CAD build for the part. Positions are in the model's coordinates, mm. A direction names the side the tool comes from. Coordinates: 2 decimals unless noted, no trailing zeros. Loops run counter-clockwise (first coordinate to the right, second up) from the corner with the lowest first, then second, coordinate; pieces in that order, holes last. Notation, with made-up numbers: (71, 46.5) -> (128, 46.5) arc R16 cw to (128, 57.5) -> close; hole circle Ø4 at (53, -22.75). An arc over 180 degrees is marked (long way). Write item = value, one per line. Start each with the question number.
(1) Pull direction Z, two halves, no side cores. Call faces 1 (the face through (-5.95, 4.19, -0.13)), 2 (the face through (39.1, 2.5, 13.5)), 3 (the face through (36, 2, 15)), 4 (the face through (-40, 2, 19)): +Z half, -Z half, draft (parallel to the pull), parting line (faces both ways), or undercut.
(2) Band-saw the part on C-C (x = -40). Write the cut outline in (y, z).
(3) Flat gauge pins, fed straight in: P1, Ø3, axis at x = -5.5, y = 4, coming from the +Z side; P2, Ø4.5, axis at x = 40, z = 15, coming from the +Y side; P3, Ø5, axis at x = -2, z = 2.5, coming from the +Y side. Where does each tip first touch, or does it go through?
(4) Band-saw the part on A-A (x = 40). Write the cut outline in (y, z), and give its area (3 significant figures).
(5) Band-saw the part on D-D (z = 0). Write the cut outline in (x, y), and give its area (3 significant figures).
(6) Band-saw the part on B-B (z = 15). Write the cut outline in (x, y), and give its area (3 significant figures).
(7) Tool access for faces 5 (the face through (42, 5, 15)), 6 (the face through (-29.4, 3.5, 0.1)), 7 (the face through (-36, 2, -15)): list every direction of +Z, -Z, +X, -X, +Y, -Y with a clear straight run to the whole face (end or side of a thin tool).
(8) Drill centre lines: line 1 (Z direction, x = 40, y = 1.15); line 2 (X direction, y = 4.25, z = -15.5); line 3 (X direction, y = 1.25, z = 12.5). Where is each one in solid material? Low to high. Write a range as from..to.
Autodesk Inventor part; units mm, degrees
ref_plane "YZ Plane" through (0, 0, 0) normal (1, 0, 0) x (0, 1, 0)
ref_plane "XZ Plane" through (0, 0, 0) normal (0, 1, 0) x (-1, 0, 0)
ref_plane "XY Plane" through (0, 0, 0) normal (0, 0, 1) x (1, 0, 0)
sketch "Sketch1" plane through (0, 0, 0) normal (0, 1, 0) x (-1, 0, 0)
  line L0 (44, 11) -> (-44, 11)
  line L1 (-44, 11) -> (-44, -11)
  line L2 (-44, -11) -> (44, -11)
  line L3 (44, -11) -> (44, 11)
  line L4 (44, 11) -> (-44, -11) construction
  line L5 (-44, 11) -> (44, -11) construction
  line L6 (36, 19) -> (44, 19)
  line L7 (44, 19) -> (44, 11)
  line L8 (44, 11) -> (36, 11)
  line L9 (36, 11) -> (36, 19)
  line L10 (36, 19) -> (44, 11) construction
  line L11 (44, 19) -> (36, 11) construction
  line L12 (36, -19) -> (44, -19)
  line L13 (44, -19) -> (44, -11)
  line L14 (44, -11) -> (36, -11)
  line L15 (36, -11) -> (36, -19)
  line L16 (36, -19) -> (44, -11) construction
  line L17 (44, -19) -> (36, -11) construction
  line L18 (-36, 19) -> (-44, 19)
  line L19 (-44, 19) -> (-44, 11)
  line L20 (-44, 11) -> (-36, 11)
  line L21 (-36, 11) -> (-36, 19)
  line L22 (-36, 19) -> (-44, 11) construction
  line L23 (-44, 19) -> (-36, 11) construction
  line L24 (-36, -19) -> (-44, -19)
  line L25 (-44, -19) -> (-44, -11)
  line L26 (-44, -11) -> (-36, -11)
  line L27 (-36, -11) -> (-36, -19)
  line L28 (-36, -19) -> (-44, -11) construction
  line L29 (-44, -19) -> (-36, -11) construction
  circle A0 centre (40, 15) radius 1.75
  circle A1 centre (40, -15) radius 1.75
  circle A2 centre (-40, 15) radius 1.75
  circle A3 centre (-40, -15) radius 1.75
  point P0 (0, 0)
  dimension "d0" = 22
  dimension "d1" = 88
  dimension "d2" = 8
  dimension "d3" = 8
  dimension "d8" = 3.5
  dimension "d9" = 3.5
  dimension "d10" = 3.5
  dimension "d11" = 3.5
  dimension "d24" = 30
  dimension "d25" = 80
extrude "Extrusion1" add sketch "Sketch1" along normal blind 10 contours L3 L2 L1 L0
extrude "Extrusion2" add sketch "Sketch1" along normal blind 5 contours L0 L9 L6 L7 | L13 L12 L15 L2 | L0 L19 L18 L21 | L27 L24 L25 L2
sketch "Sketch3" plane through (0, 10, 0) normal (0, 1, 0) x (1, 0, 0)
  line L0 (44, 11) -> (44, 19)
  line L1 (-44, -11) -> (44, -11)
  line L2 (44, -11) -> (44, 11)
  line L3 (44, 11) -> (-44, 11)
  line L4 (-44, 11) -> (-44, -11)
  line L5 (-44, -11) -> (44, 11) construction
  line L6 (44, -11) -> (-44, 11) construction
  line L7 (-36, -19) -> (-36, -11)
  line L8 (-44, -11) -> (-36, -11)
  line L9 (-44, -11) -> (-44, -19)
  line L10 (-44, -19) -> (-36, -19)
  circle A0 centre (-40, -15) radius 1.75
  line L11 (-36, 11) -> (-44, 11)
  line L12 (-36, 11) -> (-36, 19)
  line L13 (-36, 19) -> (-44, 19)
  line L14 (-44, 19) -> (-44, 11)
  circle A1 centre (-40, 15) radius 1.75
  line L15 (36, 19) -> (36, 11)
  line L16 (44, 11) -> (36, 11)
  line L17 (44, 11) -> (44, 19)
  line L18 (44, 19) -> (36, 19)
  circle A2 centre (40, 15) radius 1.75
  line L19 (36, -11) -> (44, -11)
  line L20 (36, -11) -> (36, -19)
  line L21 (36, -19) -> (44, -19)
  line L22 (44, -19) -> (44, -11)
  circle A3 centre (40, -15) radius 1.75
  point P0 (0, 0)
sketch "Sketch2" plane through (0, 10, 0) normal (0, 1, 0) x (1, 0, 0)
  line L0 (-98.02, 0) -> (97.5, 0)
  line L1 (-39, 5) -> (-39, 6.5)
  line L2 (-39, 6.5) -> (-20, 6.5)
  line L3 (-20, 6.5) -> (8.5, 5.1)
  line L4 (8.5, 5.1) -> (24.3, 5.1)
  line L5 (24.3, 5.1) -> (24.3, 5.6)
  line L6 (24.3, 5.6) -> (25.3, 6.1)
  line L7 (25.3, 6.1) -> (37.5, 6.1)
  line L8 (37.5, 6.1) -> (37.5, 0)
  line L9 (-38.5, 0) -> (37.5, 0)
  line L10 (-44, 11) -> (-44, -11)
  line L11 (-39, 5) -> (-44, 5)
  line L12 (-44, 5) -> (-44, 0)
  point P0 (0, 0)
  dimension "d12" = 13
  dimension "d13" = 12.2
  dimension "d14" = 1
  dimension "d15" = 0.5
  dimension "d16" = 10.2
  dimension "d17" = 76.5
  dimension "d18" = 13.2
  dimension "d19" = 19
  dimension "d20" = 5
  dimension "d21" = 29
  dimension "d23" = 10
revolve "Revolution1" cut sketch "Sketch2" angle 360 about axis through (-98.02, 10, 0) along (1, 0, 0)
equation "\"d9\" = d8"
equation "\"d10\" = d8"
equation "\"d11\" = d8"
properties part number "stick_antenna_case"
Findings below:
q1.face_1 = undercut
q1.face_2 = undercut
q1.face_3 = draft
q1.face_4 = +Z half
q2.outline = (0, -19) -> (5, -19) -> (5, -16.75) -> (0, -16.75) -> close; (0, -13.25) -> (5, -13.25) -> (5, -11) -> (10, -11) -> (10, -5) arc R5 cw to (10, 5) -> (10, 11) -> (5, 11) -> (5, 13.25) -> (0, 13.25) -> close; (0, 16.75) -> (5, 16.75) -> (5, 19) -> (0, 19) -> close
q3.P1 = 11
q3.P2 = 5
q3.P3 = 7.45
q4.outline = (0, -19) -> (5, -19) -> (5, -16.75) -> (0, -16.75) -> close; (0, -13.25) -> (5, -13.25) -> (5, -11) -> (10, -11) -> (10, 11) -> (5, 11) -> (5, 13.25) -> (0, 13.25) -> close; (0, 16.75) -> (5, 16.75) -> (5, 19) -> (0, 19) -> close
q4.area = 265 mm²
q5.outline = (-44, 0) -> (44, 0) -> (44, 10) -> (37.5, 10) -> (37.5, 3.9) -> (25.3, 3.9) -> (24.3, 4.4) -> (24.3, 4.9) -> (8.5, 4.9) -> (-20, 3.5) -> (-39, 3.5) -> (-39, 5) -> (-44, 5) -> close
q5.area = 405 mm²
q6.outline = (-44, 0) -> (-41.75, 0) -> (-41.75, 5) -> (-44, 5) -> close; (-38.25, 0) -> (-36, 0) -> (-36, 5) -> (-38.25, 5) -> close; (36, 0) -> (38.25, 0) -> (38.25, 5) -> (36, 5) -> close; (41.75, 0) -> (44, 0) -> (44, 5) -> (41.75, 5) -> close
q6.area = 45.0 mm²
q7.face_5 = +Z, +X, -X, +Y
q7.face_6 = +Y
q7.face_7 = -Z, +Y, -Y
q8.line_1 = -19..-16.75, -13.25..13.25, 16.75..19
q8.line_2 = -44..-41.68, -38.32..-36, 36..38.32, 41.68..44
q8.line_3 = -44..-36, 36..44
